Autodesk Inventor part; units mm, degrees
ref_plane "Work Plane2" through (-10.8195, -5.0452, 0) normal (0.9063, 0.4226, 0) x (-0.4226, 0.9063, 0)
ref_plane "XZ Plane" through (0, 0, 0) normal (0, 1, 0) x (-1, 0, 0)
ref_plane "XY Plane" through (0, 0, 0) normal (0, 0, 1) x (1, 0, 0)
sketch "Sketch1" plane through (0, 0, 0) normal (0, 0, 1) x (1, 0, 0)
  circle A0 centre (0, 0) radius 11.938
  dimension "d0" = 23.876
extrude "Extrusion1" add sketch "Sketch1" along normal blind 12.7
sketch "Sketch3" plane through (0, 0, 0) normal (0, 0, -1) x (-1, 0, 0)
  circle A0 centre (8.89, 0) radius 1.27
  circle A1 centre (0, 8.89) radius 1.27
  circle A2 centre (-8.89, 0) radius 1.27
  circle A3 centre (0, -8.89) radius 1.27
  point P0 (0, 0)
  dimension "d3" = 2.54
  dimension "d4" = 8.89
  dimension "d7" = 360
extrude "Extrusion2" cut sketch "Sketch3" against normal through all
sketch "Sketch4" plane through (0, 0, 12.7) normal (0, 0, 1) x (1, 0, 0)
  line L0 (4.6745, 1.2525) -> (3.4219, -3.4219)
  line L1 (3.4219, -3.4219) -> (-1.2525, -4.6745)
  line L2 (-1.2525, -4.6745) -> (-4.6745, -1.2525)
  line L3 (-4.6745, -1.2525) -> (-3.4219, 3.4219)
  line L4 (-3.4219, 3.4219) -> (1.2525, 4.6745)
  line L5 (1.2525, 4.6745) -> (4.6745, 1.2525)
  circle A0 centre (8.89, 0) radius 1.27
  circle A1 centre (-8.89, 0) radius 1.27
  circle A2 centre (0, 8.89) radius 1.27
  circle A3 centre (0, -8.89) radius 1.27
  circle A4 centre (0, 0) radius 11.938
  line L6 (-2.9635, -2.9635) -> (-8.4414, -8.4414) construction
  circle A5 centre (0, 0) radius 11.938 construction
  line L7 (-8.89, 0) -> (-8.4414, -8.4414) construction
  line L8 (0, -8.89) -> (-8.4414, -8.4414) construction
  dimension "d11" = 8.382
extrude "Extrusion3" cut sketch "Sketch4" against normal blind 7.62 contours L0 L1 L2 L3 L4 L5
sketch "Sketch5" plane through (0, 0, 0) normal (0, 0, -1) x (-1, 0, 0)
  circle A0 centre (0, 0) radius 3.048
  dimension "d14" = 6.096
extrude "Extrusion4" cut sketch "Sketch5" against normal through all
sketch "Sketch7" plane through (-1.2525, -4.6745, 5.08) normal (0.7071, 0.7071, 0) x (-0.7071, 0.7071, 0)
  circle A0 centre (2.4197, 3.556) radius 1.27
  line L0 (14.3577, 7.62) -> (-9.5183, 7.62)
  line L1 (13.5978, 7.62) -> (13.5978, -5.08) construction
  line L2 (13.5978, -5.08) -> (-8.7585, -5.08) construction
  line L3 (-8.7585, -5.08) -> (-8.7585, 7.62) construction
  line L4 (-8.7585, 7.62) -> (0, 7.62) construction
  line L5 (0, 7.62) -> (4.8393, 7.62) construction
  line L6 (4.8393, 7.62) -> (13.5978, 7.62) construction
  line L7 (0, 7.62) -> (0, 0) construction
  line L8 (0, 0) -> (4.8393, 0) construction
  line L9 (4.8393, 0) -> (4.8393, 7.62) construction
  line L10 (13.5978, 7.62) -> (2.4197, 3.556) construction
  line L11 (2.4197, 3.556) -> (-8.7585, 7.62) construction
  point P0 (2.4197, -5.08)
  dimension "d22" = 4.064
  dimension "d39" = 2.54
extrude "Extrusion6" cut sketch "Sketch7" against normal through all
sketch "Sketch8" plane through (0, 0, 0) normal (0, 0, -1) x (-1, 0, 0)
  circle A0 centre (0, 0) radius 4.064
  dimension "d25" = 8.128
extrude "Extrusion7" cut sketch "Sketch8" against normal blind 0.889
chamfer "Chamfer1" distance 1.016 angle 45 1 edges at (3.048, 0, 0.889)
ref_plane "Work Plane2" through (-10.8195, -5.0452, 0) normal (0.9063, 0.4226, 0) x (-0.4226, 0.9063, 0)
ref_plane "Work Plane1" through (0, 0, 0) normal (0.9063, 0.4226, 0) x (0, 0, 1)
sketch "Sketch9" plane through (-10.8195, -5.0452, 0) normal (0.9063, 0.4226, 0) x (-0.4226, 0.9063, 0)
  circle A0 centre (0, 8.128) radius 1.7145
  line L0 (11.938, 12.7) -> (-11.938, 12.7)
  point P0 (0, 0)
  dimension "d32" = 3.429
  dimension "d33" = 4.572
extrude "Extrusion8" cut sketch "Sketch9" along normal blind 1.905
pattern_circular "Circular Pattern1" count 4 over 360 about axis through (0, 0, 0) along (0, 0, 1) of "Extrusion8"
properties part number "HexNutShaftServoCoupler" material "ABS Plastic"
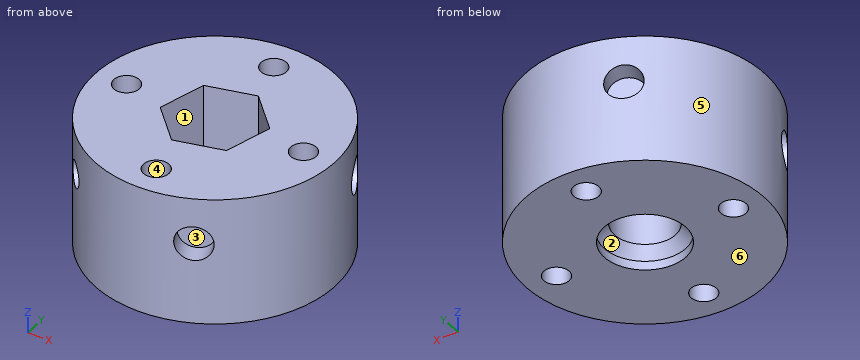
Could you check a few things on this model? Use its own coordinates, in mm. Face numbers are marked on the shaded views. A direction names the side the tool comes from. Coordinates: 2 decimals unless noted, no trailing zeros. Write each loop counter-clockwise with the first axis right and the second up, starting at its lowest first coordinate (ties: lowest second). Pieces come first, ordered by that corner, then holes. Notation, with made-up numbers: M -30.75,-21.5 L 6.25,-21.5 A11 ccw 6.25,-14.5 Z; hole C -8.5,-25 d4. An arc over 180 degrees is marked long. One line per question, with ' | ' between items.
1) For the marked faces 1, 2 and 3, which set-ups out of +Z, -Z, +X, -X, +Y, -Y let a thin tool reach every point of the face, with its end or its side?
Checks:
face 1: +Z | face 2: -Z | face 3: none
2) If we mould it in two halves opening along Y, with no side actions, what happens to the marked faces 4, 5 and 6? For each: released by +Y, released by -Y, zero draft, split by the parting line, or undercut.
Checks:
face 4: undercut | face 5: split by the parting line | face 6: zero draft
3) Imagine slicing it at A-A, the plane y = 0. Give the number of separate pieces and of enclosed holes in the cut face, and give its area (3 significant figures).
Checks:
separate pieces: 4 | enclosed holes: 0 | area: 139 mm²
4) Imagine slicing it at B-B, the plane z = 7. Write out the boundary of the cut face in (x, y).
Checks:
outline: M -11.3,-3.85 L -9.64,-3.07 L -8.55,-5.41 L -10.21,-6.19 A11.94 ccw 3.85,-11.3 L 3.07,-9.64 L 5.41,-8.55 L 6.19,-10.21 A11.94 ccw 11.3,3.85 L 9.64,3.07 L 8.55,5.41 L 10.21,6.19 A11.94 ccw -3.85,11.3 L -3.07,9.64 L -5.41,8.55 L -6.19,10.21 A11.94 ccw Z; hole C -8.89,0 d2.54; hole M -4.67,-1.25 L -1.25,-4.67 L 3.42,-3.42 L 4.67,1.25 L 1.25,4.67 L -3.42,3.42 Z; hole C 0,-8.89 d2.54; hole C 0,8.89 d2.54; hole C 8.89,0 d2.54
5) I need wall thicknesses on probe 1 along Y at (x, z) = (0, 0.2); probe 2 along Y at (x, z) = (0, 3.5); probe 3 along Y at (x, z) = (2.75, 8). Which ranges of each line are inside material? Lowest first, please. Write a range as [from, to].
Checks:
probe 1: [-11.94, -10.16], [-7.62, -4.06], [4.06, 7.62], [10.16, 11.94] | probe 2: [-11.94, -10.16], [-7.62, -3.05], [3.05, 7.62], [10.16, 11.94] | probe 3: [-11.62, -9.94], [-9.79, -3.6], [3.18, 11.62]
6) For pin 1 Ø1 at (y, z) = (4.5, 5.5) entering from -X; pin 2 Ø12 at (x, y) = (-2, -6) entering from -Z; pin 3 Ø2 at (y, z) = (8, 2.5) entering from +X; pin 4 Ø1.5 at (x, z) = (8, 11) entering from +Y, each with a flat end and sliding along its axis, tell me the tip position at first contact or that it passes through.
Checks:
pin 1: x = -11.25 | pin 2: z = 0 | pin 3: x = 9.67 | pin 4: y = 9.48
